Answer from the drawing. Dimensions are ordinates in mm from the lowest x, y and z of the part. Give positions to 0.01 mm unless a question says otherwise; leave off trailing zeros. Loops run counter-clockwise (first coordinate to the right, second up) from the corner with the lowest first, then second, coordinate; pieces in that order, holes last. Notation, with made-up numbers: M 72,2 L 90,2 A17 ccw 90,21 Z; hole C -19,-6.75 d8. An arc over 180 degrees is marked long. Use a Markdown table: item, result.
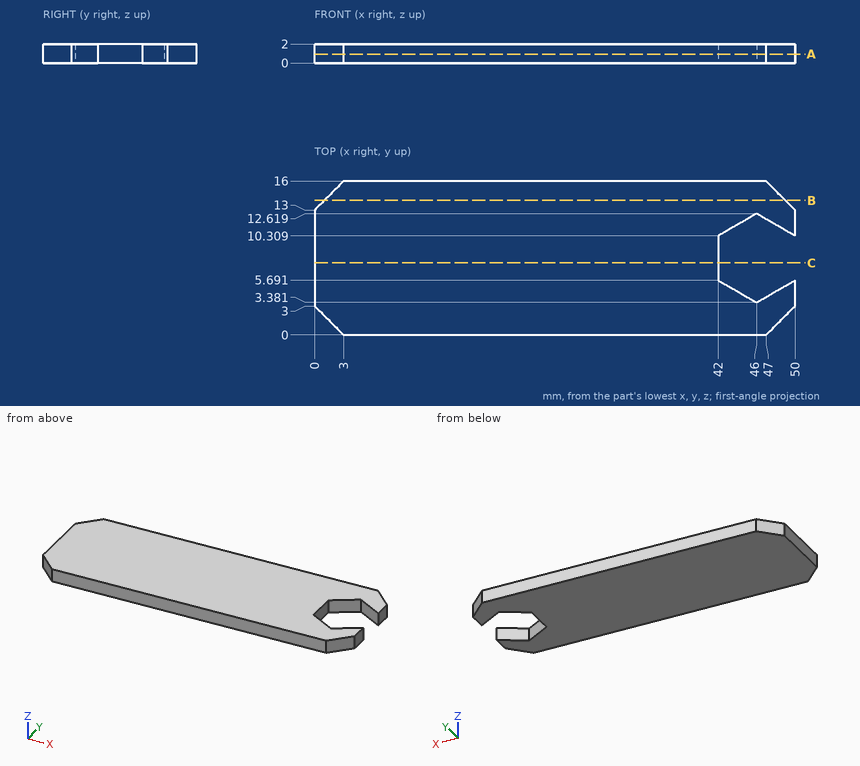
(1) Consider probe 1 along Y at (x, z) = (46, 1.5); probe 2 along X at (y, z) = (4.5, 0.7) (1 decimal); probe 3 along X at (y, z) = (8, 1.45). Determine where each line is inside the solid, lowest interval first. Write a range as [from, to].
Entries:
| item | result |
|---|---|
| probe 1 | y = [0, 3.38], [12.62, 16] |
| probe 2 | x = [0, 44.1], [47.9, 50] |
| probe 3 | x = [0, 42] |
(2) A cutting plane is placed at C-C (y = 7.5). Write down the section's boundary in (x, z).
Entries:
| item | result |
|---|---|
| outline | M 0,0 L 42,0 L 42,2 L 0,2 Z |
(3) A cutting plane is placed at A-A (z = 0.95). Write down the section's boundary in (x, y).
Entries:
| item | result |
|---|---|
| outline | M 0,3 L 3,0 L 47,0 L 50,3 L 50,5.69 L 46,3.38 L 42,5.69 L 42,10.31 L 46,12.62 L 50,10.31 L 50,13 L 47,16 L 3,16 L 0,13 Z |
(4) A cutting plane is placed at B-B (y = 14). Write down the section's boundary in (x, z).
Entries:
| item | result |
|---|---|
| outline | M 1,0 L 49,0 L 49,2 L 1,2 Z |
